Drawing for the job (mm, zero at the part's lowest x, y, z). Round coordinates to 2 decimals unless told otherwise and drop trailing zeros. Order: outer loops, then holes, each group sorted by start corner. A loop starts at its lowest first (then second) coordinate and runs counter-clockwise, first axis right, second up. Notation, with made-up numbers: (36, 80.5) - (65, 80.5) arc R13 cw to (65, 89.5) - close; hole circle Ø9 at (52.5, -36). An arc over 180 degrees is marked (long way). Put each result on its own line as item: value. Start each with the question number.
Item 1: Saw through at A-A on x = 384.5. List the corners of the cut face in (y, z).
Item 2: Probe probe 1 along Y at (x, z) = (397, 4.5); probe 2 along X at (y, z) = (167.5, 19.5) (3 decimals); probe 3 along Y at (x, z) = (347.5, 7.5). List the from-to ranges inside material, lowest first.
Item 3: Pin check, flat tips, straight feed: pin 1 Ø10 at (y, z) = (362, 21.5) entering from +X (3 decimals); pin 2 Ø2 at (y, z) = (234.5, 5.5) entering from -X (3 decimals); pin 3 Ø12.5 at (x, z) = (72.5, 14) entering from -Y; pin 4 Ø12 at (y, z) = (527.5, 7.5) entering from -X. Stop position of each tip, or through.
Item 4: Saw through at C-C on y = 133. List the corners of the cut face in (x, z) (3 decimals), plus the area to 4 significant figures.
Item 5: Saw through at B-B on z = 6. List the corners of the cut face in (x, y) (3 decimals), plus the area to 3 significant figures.
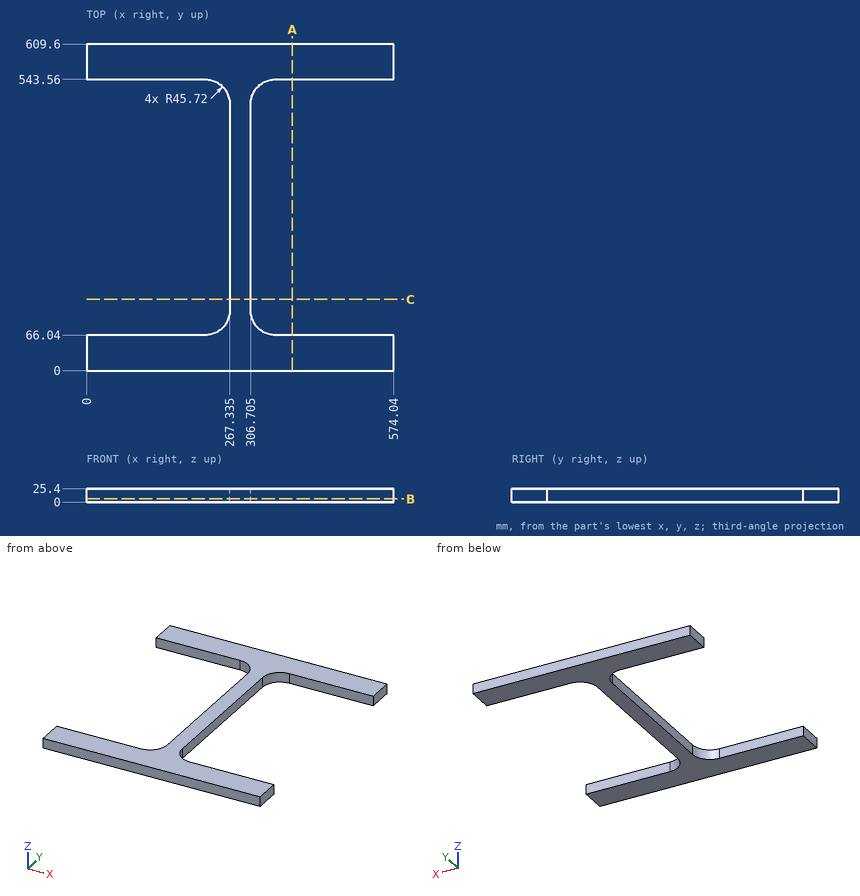
Results found:
1. outline: (0, 0) - (66.04, 0) - (66.04, 25.4) - (0, 25.4) - close; (543.56, 0) - (609.6, 0) - (609.6, 25.4) - (543.56, 25.4) - close
2. probe 1: y = 0 to 66.04, 543.56 to 609.6
2. probe 2: x = 267.335 to 306.705
2. probe 3: y = 0 to 66.31, 543.29 to 609.6
3. pin 1: stops at x = 306.705
3. pin 2: stops at x = 267.335
3. pin 3: stops at y = 0
3. pin 4: stops at x = 250.23
4. outline: (267.335, 0) - (306.705, 0) - (306.705, 25.4) - (267.335, 25.4) - close
4. area: 1,000 mm²
5. outline: (0, 0) - (574.04, 0) - (574.04, 66.04) - (352.425, 66.04) arc R45.72 cw to (306.705, 111.76) - (306.705, 497.84) arc R45.72 cw to (352.425, 543.56) - (574.04, 543.56) - (574.04, 609.6) - (0, 609.6) - (0, 543.56) - (221.615, 543.56) arc R45.72 cw to (267.335, 497.84) - (267.335, 111.76) arc R45.72 cw to (221.615, 66.04) - (0, 66.04) - close
5. area: 96,400 mm²
